```python
from build123d import *

# Parameters (mm, degrees)
CROQUIS1_R              = 10
CROQUIS1_R_2            = 5
SALIENTE_EXTRUIR1_DEPTH = 1.5
CORTAR_EXTRUIR1_REACH   = 26.15
CROQUIS2_R              = 1.2
SALIENTE_EXTRUIR2_START = 20
CROQUIS3_R              = 6.5
CROQUIS3_R_2            = 5
SALIENTE_EXTRUIR2_DEPTH = 20
CROQUIS5_R              = 1
SALIENTE_EXTRUIR3_DEPTH = 20
CROQUIS7_R              = 1.9
CORTAR_EXTRUIR3_DEPTH   = 7
CROQUIS8_R              = 6
SALIENTE_EXTRUIR4_DEPTH = 15


with BuildPart() as part:
    # Croquis1 → Saliente-Extruir1 (new body)
    with BuildSketch(Plane.XY):
        with Locations((1.467948917, 11.200668728)):
            Circle(CROQUIS1_R)
        with Locations((1.467948917, 11.200668728)):
            Circle(CROQUIS1_R_2, mode=Mode.SUBTRACT)
    extrude(amount=-SALIENTE_EXTRUIR1_DEPTH)

    # Croquis2 → Cortar-Extruir1 (cut, up to next)
    with BuildSketch(Plane.XY, mode=Mode.PRIVATE) as cortar_extruir1_sk1:
        with Locations((1.467948917, 19.200668728)):
            Circle(CROQUIS2_R)
    cortar_extruir1_tool1 = extrude(cortar_extruir1_sk1.sketch, amount=-CORTAR_EXTRUIR1_REACH, mode=Mode.PRIVATE) & part.part
    # Croquis2 → Cortar-Extruir1 (cut, up to next)
    with BuildSketch(Plane.XY, mode=Mode.PRIVATE) as cortar_extruir1_sk2:
        with Locations((7.124803167, 16.857522978)):
            Circle(CROQUIS2_R)
    cortar_extruir1_tool2 = extrude(cortar_extruir1_sk2.sketch, amount=-CORTAR_EXTRUIR1_REACH, mode=Mode.PRIVATE) & part.part
    # Croquis2 → Cortar-Extruir1 (cut, up to next)
    with BuildSketch(Plane.XY, mode=Mode.PRIVATE) as cortar_extruir1_sk3:
        with Locations((9.467948917, 11.200668728)):
            Circle(CROQUIS2_R)
    cortar_extruir1_tool3 = extrude(cortar_extruir1_sk3.sketch, amount=-CORTAR_EXTRUIR1_REACH, mode=Mode.PRIVATE) & part.part
    # Croquis2 → Cortar-Extruir1 (cut, up to next)
    with BuildSketch(Plane.XY, mode=Mode.PRIVATE) as cortar_extruir1_sk4:
        with Locations((7.124803167, 5.543814479)):
            Circle(CROQUIS2_R)
    cortar_extruir1_tool4 = extrude(cortar_extruir1_sk4.sketch, amount=-CORTAR_EXTRUIR1_REACH, mode=Mode.PRIVATE) & part.part
    # Croquis2 → Cortar-Extruir1 (cut, up to next)
    with BuildSketch(Plane.XY, mode=Mode.PRIVATE) as cortar_extruir1_sk5:
        with Locations((1.467948917, 3.200668728)):
            Circle(CROQUIS2_R)
    cortar_extruir1_tool5 = extrude(cortar_extruir1_sk5.sketch, amount=-CORTAR_EXTRUIR1_REACH, mode=Mode.PRIVATE) & part.part
    # Croquis2 → Cortar-Extruir1 (cut, up to next)
    with BuildSketch(Plane.XY, mode=Mode.PRIVATE) as cortar_extruir1_sk6:
        with Locations((-4.188905332, 5.543814479)):
            Circle(CROQUIS2_R)
    cortar_extruir1_tool6 = extrude(cortar_extruir1_sk6.sketch, amount=-CORTAR_EXTRUIR1_REACH, mode=Mode.PRIVATE) & part.part
    # Croquis2 → Cortar-Extruir1 (cut, up to next)
    with BuildSketch(Plane.XY, mode=Mode.PRIVATE) as cortar_extruir1_sk7:
        with Locations((-6.532051083, 11.200668728)):
            Circle(CROQUIS2_R)
    cortar_extruir1_tool7 = extrude(cortar_extruir1_sk7.sketch, amount=-CORTAR_EXTRUIR1_REACH, mode=Mode.PRIVATE) & part.part
    # Croquis2 → Cortar-Extruir1 (cut, up to next)
    with BuildSketch(Plane.XY, mode=Mode.PRIVATE) as cortar_extruir1_sk8:
        with Locations((-4.188905332, 16.857522978)):
            Circle(CROQUIS2_R)
    cortar_extruir1_tool8 = extrude(cortar_extruir1_sk8.sketch, amount=-CORTAR_EXTRUIR1_REACH, mode=Mode.PRIVATE) & part.part
    add(cortar_extruir1_tool1.solids().sort_by_distance((1.467949, 19.200669, 0))[0], mode=Mode.SUBTRACT)
    add(cortar_extruir1_tool2.solids().sort_by_distance((7.124803, 16.857523, 0))[0], mode=Mode.SUBTRACT)
    add(cortar_extruir1_tool3.solids().sort_by_distance((9.467949, 11.200669, 0))[0], mode=Mode.SUBTRACT)
    add(cortar_extruir1_tool4.solids().sort_by_distance((7.124803, 5.543814, 0))[0], mode=Mode.SUBTRACT)
    add(cortar_extruir1_tool5.solids().sort_by_distance((1.467949, 3.200669, 0))[0], mode=Mode.SUBTRACT)
    add(cortar_extruir1_tool6.solids().sort_by_distance((-4.188905, 5.543814, 0))[0], mode=Mode.SUBTRACT)
    add(cortar_extruir1_tool7.solids().sort_by_distance((-6.532051, 11.200669, 0))[0], mode=Mode.SUBTRACT)
    add(cortar_extruir1_tool8.solids().sort_by_distance((-4.188905, 16.857523, 0))[0], mode=Mode.SUBTRACT)

    # Croquis3 → Saliente-Extruir2 (add)
    with BuildSketch(Plane.XY.offset(SALIENTE_EXTRUIR2_START)):
        with Locations((1.467948917, 11.200668728)):
            Circle(CROQUIS3_R)
        with Locations((1.467948917, 11.200668728)):
            Circle(CROQUIS3_R_2, mode=Mode.SUBTRACT)
    extrude(amount=-SALIENTE_EXTRUIR2_DEPTH)

    # Croquis5 → Saliente-Extruir3 (add)
    with BuildSketch(Plane.XY.offset(20)):
        with Locations((3.955391227, 17.20588569)):
            Circle(CROQUIS5_R)
        with Locations((7.473165878, 13.688111039)):
            Circle(CROQUIS5_R)
        with Locations((7.473165878, 8.713226418)):
            Circle(CROQUIS5_R)
        with Locations((3.955391227, 5.195451767)):
            Circle(CROQUIS5_R)
        with Locations((-1.019493393, 5.195451767)):
            Circle(CROQUIS5_R)
        with Locations((-4.537268044, 8.713226418)):
            Circle(CROQUIS5_R)
        with Locations((-4.537268044, 13.688111039)):
            Circle(CROQUIS5_R)
        with Locations((-1.019493393, 17.20588569)):
            Circle(CROQUIS5_R)
    extrude(amount=-SALIENTE_EXTRUIR3_DEPTH)

    # Croquis7 → Cortar-Extruir3 (cut)
    with BuildSketch(Plane.XY):
        with Locations((-4.188905332, 16.857522978)):
            Circle(CROQUIS7_R)
        with Locations((1.467948917, 19.200668728)):
            Circle(CROQUIS7_R)
        with Locations((7.124803167, 16.857522978)):
            Circle(CROQUIS7_R)
        with Locations((9.467948917, 11.200668728)):
            Circle(CROQUIS7_R)
        with Locations((7.124803167, 5.543814479)):
            Circle(CROQUIS7_R)
        with Locations((1.467948917, 3.200668728)):
            Circle(CROQUIS7_R)
        with Locations((-4.188905332, 5.543814479)):
            Circle(CROQUIS7_R)
        with Locations((-6.532051083, 11.200668728)):
            Circle(CROQUIS7_R)
    extrude(amount=CORTAR_EXTRUIR3_DEPTH, mode=Mode.SUBTRACT)

    # Croquis8 → Saliente-Extruir4 (add)
    with BuildSketch(Plane.XY.offset(20)):
        with Locations((1.467948917, 11.200668728)):
            Circle(CROQUIS8_R)
    extrude(amount=-SALIENTE_EXTRUIR4_DEPTH)


solid = part.part
```
The listing builds one solid part. Answer for the finished solid, in the listing's coordinates (mm). A direction names the side the tool comes from. Give positions to 0.01 mm unless a question says otherwise; leave off trailing zeros. Order: outer loops, then holes, each group sorted by start corner. A loop starts at its lowest first (then second) coordinate and runs counter-clockwise, first axis right, second up. Notation, with made-up numbers: (73.25, 68.25) -> (114.25, 68.25) arc R16 ccw to (114.25, 87.25) -> close; hole circle Ø5 at (39, 35.25). An arc over 180 degrees is marked (long way). Answer as a JSON object with one key per item and string values. Group by question number.
Item 1: Determine the mould class of faces 6 (the flat face through (4, 16, -1.5)), 7 (the flat face through (-3, 6.7, 7)), 8 (the flat face through (5.95, 15.63, 7)), 9 (the cylindrical face through (1.5, 17.7, 12.4)) for opening direction Z: pulls with the +Z half, pulls with the -Z half, needs draft (parallel to the pull), parting line crosses it, or undercut.
Item 2: The part is cut by section C-C on y = 10.75. Write down the section's boundary in (x, z).
Item 3: Consider L1, parallel to Z at x = 0, y = 14; L2, parallel to X at y = 17.25, z = 10.75; L3, parallel to Z at x = 9.5, y = 6.5. Determine where each line is inside the solid, lowest interval first. Write a range as from..to.
Item 4: The part is cut by section D-D on z = 16.5. Write down the section's boundary in (x, y), and give its area (3 significant figures).
Item 5: The part is cut by section A-A on y = 19.75. Write down the section's boundary in (x, z).
Item 6: Flat-ended cylindrical pins translate along their axes: pin 1 (8 mm diameter, centred on y = 9, z = 15.5, fed in from -X); pin 2 (6 mm diameter, centred on x = 1, z = 15.5, fed in from +Y); pin 3 (1 mm diameter, centred on x = 5.5, y = 19, fed in from +Z). Find the tip coordinate at first contact, or state that the pin passes through.
Item 7: The part is cut by section B-B on x = 9. Write down the section's boundary in (y, z).
Item 8: A tool of negligible diameter and unlimited length cuts with its end or side. For faces 1 (the cylindrical face through (0.38, 6.32, 1.8)), 2 (the cylindrical face through (-4.632, 11.185, 3.451)), 3 (the cylindrical face through (7.968, 11.179, 12.362)), 4 (the cylindrical face through (1.5, 17.3, 3.5)), 5 (the cylindrical face through (-2.86, 15.5, 3.45)), from which of +Z, -Z, +X, -X, +Y, -Y can it reach the whole face along a straight path? Write none if from no direction.
Result set:
{
 "1": {"face 6": "pulls with the -Z half", "face 7": "undercut", "face 8": "undercut", "face 9": "needs draft"},
 "2": {"outline": "(-8.52, -1.5) -> (-7.64, -1.5) -> (-7.64, 0) -> (-8.52, 0) -> close; (-5.42, -1.5) -> (-3.51, -1.5) -> (-3.51, 5) -> (6.45, 5) -> (6.45, -1.5) -> (8.36, -1.5) -> (8.36, 0) -> (7.62, 0) -> (7.62, 7) -> (7.95, 7) -> (7.95, 20) -> (-5.02, 20) -> (-5.02, 7) -> (-4.69, 7) -> (-4.69, 0) -> (-5.42, 0) -> close; (10.58, -1.5) -> (11.46, -1.5) -> (11.46, 0) -> (10.58, 0) -> close"},
 "3": {"L1": "5..20", "L2": "-2.02..4.95", "L3": "-1.5..0"},
 "4": {"outline": "(-4.85, 9.66) arc R1 ccw (long way) to (-4.08, 7.82) arc R6.5 ccw to (-1.91, 5.65) arc R1 ccw (long way) to (-0.07, 4.88) arc R6.5 ccw to (3, 4.88) arc R1 ccw (long way) to (4.85, 5.65) arc R6.5 ccw to (7.02, 7.82) arc R1 ccw (long way) to (7.78, 9.66) arc R6.5 ccw to (7.78, 12.74) arc R1 ccw (long way) to (7.02, 14.58) arc R6.5 ccw to (4.85, 16.75) arc R1 ccw (long way) to (3, 17.52) arc R6.5 ccw to (-0.07, 17.52) arc R1 ccw (long way) to (-1.91, 16.75) arc R6.5 ccw to (-4.08, 14.58) arc R1 ccw (long way) to (-4.85, 12.74) arc R6.5 ccw to start", "area": "146 mm²"},
 "5": {"outline": "(-3.72, -1.5) -> (0.4, -1.5) -> (0.4, 0) -> (-3.72, 0) -> close; (2.53, -1.5) -> (6.66, -1.5) -> (6.66, 0) -> (2.53, 0) -> close"},
 "6": {"pin 1": "x = -5.54", "pin 2": "y = 18.21", "pin 3": "z = 0"},
 "7": {"outline": "(4.62, -1.5) -> (10.1, -1.5) -> (10.1, 0) -> (4.62, 0) -> close; (12.31, -1.5) -> (17.78, -1.5) -> (17.78, 0) -> (12.31, 0) -> close"},
 "8": {"face 1": "-Z", "face 2": "-X", "face 3": "+Z, +X", "face 4": "+Y", "face 5": "-X, +Y"}
}
